from build123d import *

# Parameters (mm, degrees)
SKETCH1_W                                 = 175.514
SKETCH1_H                                 = 35.5092
BOSS_EXTRUDE1_DEPTH                       = 1.0668
CUT_EXTRUDE2_DEPTH                        = 177.412947596
SKETCH8_W                                 = 6.7056
SKETCH8_H                                 = 6.5278
SKETCH8_W_2                               = 6.35
SKETCH8_H_2                               = 6.1722
SKETCH8_W_3                               = 1.0668
SKETCH8_H_3                               = 6.35
CUT_EXTRUDE3_DEPTH                        = 90.541358781
CSK_FOR_6_FLAT_HEAD_MACHINE_SCREW_2_COUNT = 2
CSK_FOR_6_FLAT_HEAD_MACHINE_SCREW_2_PITCH = 24.166931253
CSK_FOR_6_FLAT_HEAD_MACHINE_SCREW_3_COUNT = 2
CSK_FOR_6_FLAT_HEAD_MACHINE_SCREW_3_PITCH = 27.386313674
CSK_FOR_6_FLAT_HEAD_MACHINE_SCREW_4_COUNT = 2
CSK_FOR_6_FLAT_HEAD_MACHINE_SCREW_4_PITCH = 118.84025
CSK_FOR_6_FLAT_HEAD_MACHINE_SCREW_5_COUNT = 2
CSK_FOR_6_FLAT_HEAD_MACHINE_SCREW_5_PITCH = 142.976487796
CSK_FOR_6_FLAT_HEAD_MACHINE_SCREW_6_COUNT = 2
CSK_FOR_6_FLAT_HEAD_MACHINE_SCREW_6_PITCH = 143.555722815


with BuildPart() as part:
    # Sketch1 → Boss-Extrude1 (new body)
    with BuildSketch(Plane.XY):
        Rectangle(SKETCH1_W, SKETCH1_H)
    extrude(amount=BOSS_EXTRUDE1_DEPTH)

    # Sketch7 → Cut-Extrude2 (cut, through all)
    with BuildSketch(Plane.ZY.offset(87.757)):
        Polygon((0, 17.138682733), (1.0668, 17.7546), (0, 17.7546), align=None)
        Polygon((0, -17.7546), (1.0668, -17.138682733), (1.0668, -17.7546), align=None)
    extrude(amount=-CUT_EXTRUDE2_DEPTH, mode=Mode.SUBTRACT)

    # Sketch8 → Cut-Extrude3 (cut, through all)
    # profile 1 of 4: a face of its own
    with BuildSketch(Plane(origin=(0, 0, 0), x_dir=(-1, 0, 0), z_dir=(0, 0, -1))):
        with Locations((59.3852, -7.303463684)):
            Rectangle(SKETCH8_W, SKETCH8_H)
        with Locations((59.3852, -7.303463684)):
            Rectangle(SKETCH8_W_2, SKETCH8_H_2, mode=Mode.SUBTRACT)
    # profile 2 of 4: a face of its own
    with BuildSketch(Plane(origin=(0, 0, 0), x_dir=(-1, 0, 0), z_dir=(0, 0, -1))):
        with Locations((-87.2236, -0.494716366)):
            Rectangle(SKETCH8_W_3, SKETCH8_H_3)
    # profile 3 of 4: a face of its own
    with BuildSketch(Plane(origin=(0, 0, 0), x_dir=(-1, 0, 0), z_dir=(0, 0, -1))):
        with Locations((-59.45505, -7.303467884)):
            Rectangle(SKETCH8_W, SKETCH8_H)
        with Locations((-59.45505, -7.303467884)):
            Rectangle(SKETCH8_W_2, SKETCH8_H_2, mode=Mode.SUBTRACT)
    # profile 4 of 4: a face of its own
    with BuildSketch(Plane(origin=(0, 0, 0), x_dir=(-1, 0, 0), z_dir=(0, 0, -1))):
        with Locations((87.29345, -0.494712166)):
            Rectangle(SKETCH8_W_3, SKETCH8_H_3)
    extrude(amount=-CUT_EXTRUDE3_DEPTH, mode=Mode.SUBTRACT)


with BuildPart() as cut_extrude3_kept_piece:
    # of the separate pieces the step leaves, the one the design keeps (cut_extrude3_pieces_kept)
    add(part.part.solids().sort_by_distance((-87.757, -17.138682733, 1.0668))[0])

    # Sketch9 → CSK for #6 Flat Head Machine Screw (100)1 (revolve, cut)
    with BuildSketch(Plane(origin=(59.45505, 5.307632116, 0), x_dir=(0, 1, 0), z_dir=(1, 0, 0))):
        Polygon((0, 0), (0, 1.0668), (1.89865, 1.0668), (1.89865, 1.380025208), (3.5433, 0), align=None)
    csk_for_6_flat_head_machine_screw_100 = revolve(axis=Axis((59.45505, 5.307632116, -6.35), (0, 0, 1)), mode=Mode.SUBTRACT)

    # CSK for _6 Flat Head Machine Screw _ 2: CSK for #6 Flat Head Machine Screw (100)1 ×2
    with Locations(*[Vector(0.9984718269541709, 0.05526310504125029, 0) * (i * CSK_FOR_6_FLAT_HEAD_MACHINE_SCREW_2_PITCH) for i in range(1, CSK_FOR_6_FLAT_HEAD_MACHINE_SCREW_2_COUNT)]):
        add(csk_for_6_flat_head_machine_screw_100, mode=Mode.SUBTRACT)

    # CSK for _6 Flat Head Machine Screw _ 3: CSK for #6 Flat Head Machine Screw (100)1 ×2
    with Locations(*[Vector(0.881097043122147, -0.4729355142103514, 0) * (i * CSK_FOR_6_FLAT_HEAD_MACHINE_SCREW_3_PITCH) for i in range(1, CSK_FOR_6_FLAT_HEAD_MACHINE_SCREW_3_COUNT)]):
        add(csk_for_6_flat_head_machine_screw_100, mode=Mode.SUBTRACT)

    # CSK for _6 Flat Head Machine Screw _ 4: CSK for #6 Flat Head Machine Screw (100)1 ×2
    with Locations(*[(-i * CSK_FOR_6_FLAT_HEAD_MACHINE_SCREW_4_PITCH, 0, 0) for i in range(1, CSK_FOR_6_FLAT_HEAD_MACHINE_SCREW_4_COUNT)]):
        add(csk_for_6_flat_head_machine_screw_100, mode=Mode.SUBTRACT)

    # CSK for _6 Flat Head Machine Screw _ 5: CSK for #6 Flat Head Machine Screw (100)1 ×2
    with Locations(*[Vector(-0.9999563718759208, 0.009341003412130584, 0) * (i * CSK_FOR_6_FLAT_HEAD_MACHINE_SCREW_5_PITCH) for i in range(1, CSK_FOR_6_FLAT_HEAD_MACHINE_SCREW_5_COUNT)]):
        add(csk_for_6_flat_head_machine_screw_100, mode=Mode.SUBTRACT)

    # CSK for _6 Flat Head Machine Screw _ 6: CSK for #6 Flat Head Machine Screw (100)1 ×2
    with Locations(*[Vector(-0.9959216337502219, -0.09022249956795243, 0) * (i * CSK_FOR_6_FLAT_HEAD_MACHINE_SCREW_6_PITCH) for i in range(1, CSK_FOR_6_FLAT_HEAD_MACHINE_SCREW_6_COUNT)]):
        add(csk_for_6_flat_head_machine_screw_100, mode=Mode.SUBTRACT)


solid = cut_extrude3_kept_piece.part
Build history of the part. All positions in model axes, mm. Give positions to 0.01 mm unless a question says otherwise; leave off trailing zeros. Order: outer loops, then holes, each group sorted by start corner. A loop starts at its lowest first (then second) coordinate and runs counter-clockwise, first axis right, second up. Notation, with made-up numbers: M 79.25,-33.75 L 90.25,-33.75 A29 ccw 90.25,-10.75 Z; hole C 21.25,-26.5 d8. An arc over 180 degrees is marked long. Use one line per item in the form item = value.
1) Drop a flat-ended pin along its axis: pin 1 (0.5 mm diameter, centred on x = -59.5, z = 1, fed in from +Y). Give the stop position or say it passes through.
Calculated:
pin_1 = 17.75
2) Probe probe 1 along X at (y, z) = (-5, 1); probe 2 along Y at (x, z) = (61.5, 0.9); probe 3 along X at (y, z) = (-8, 0.85). List the from-to ranges inside material, lowest first.
Calculated:
probe_1 = -87.76 to -62.74, -56.03 to 56.1, 62.81 to 87.76
probe_2 = -17.23 to -10.57, -4.04 to 3.92, 6.69 to 17.66
probe_3 = -87.76 to -86.02, -81.01 to -62.74, -56.03 to 56.1, 62.81 to 81.08, 86.09 to 87.76
3) Saw through at B-B (x = 49.5). Give the cut face in (y, z), plus the area to 3 significant figures.
Calculated:
outline = M -17.75,0 L 17.14,0 L 17.75,1.07 L -17.14,1.07 Z
area = 37.2 mm2
4) Saw through at A-A (z = 0.35). State how many separate pieces and enclosed holes the cut face has, plus the area to 3 significant figures.
Calculated:
separate_pieces = 1
enclosed_holes = 8
area = 5,840 mm2
